```python
from build123d import *

# Parameters (mm, degrees)
F0_R      = 8.5
F1_DEPTH  = 20
F2_W      = 14.2
F2_H      = 5.2
F3_DEPTH  = 15.001
F5_DEPTH  = 15
F6_W      = 1
F6_H      = 2.6394567484
F7_DEPTH  = 20.001
F8_W      = 1.5
F8_H      = 3.5
F9_DEPTH  = 20
F11_DEPTH = 20
F13_DEPTH = 15
F15_DEPTH = 15.001
F16_R     = 3
F17_R     = 0.2
F19_DEPTH = 15


with BuildPart() as f1:
    # F0 (on Front) → F1 (new body)
    with BuildSketch(Plane.XZ):
        with BuildLine():
            Line((0, 18), (0, 0))
            Line((0, 0), (15, 0))
            Line((15, 0), (15, 9.3397459622))
            ThreePointArc((15, 9.3397459622), (15, 26.6602540378), (0, 18))
        make_face()
        with Locations((10, 18)):
            Circle(F0_R, mode=Mode.SUBTRACT)
    extrude(amount=F1_DEPTH)

    # F2 (on face) → F3 (cut, through all)
    with BuildSketch(Plane.YZ.offset(15)):
        Polygon((-3.8, 2), (-2, 2), (-2, 9), (-20, 9), (-20, 7.2), (-3.8, 7.2), align=None)
        with Locations((-12.9, 2.6)):
            Rectangle(F2_W, F2_H)
    extrude(amount=-F3_DEPTH, mode=Mode.SUBTRACT)

    # F4 (on face) → F5 (join, through all)
    with BuildSketch(Plane.YZ.offset(15)):
        Polygon((-20, 7.2), (-15.5, 7.2), (-15.5, 8), align=None)
        Polygon((-15.5, 8.2), (-15.5, 9), (-20, 9), align=None)
    extrude(amount=-F5_DEPTH)

    # F6 (on face) → F7 (cut, through all)
    with BuildSketch(Plane.XZ.offset(20)):
        with Locations((15.5, 10.6594743364)):
            Rectangle(F6_W, F6_H)
    extrude(amount=-F7_DEPTH, mode=Mode.SUBTRACT)

    # F8 (on face) → F9 (join, through all)
    with BuildSketch(Plane.XZ.offset(20)):
        with Locations((14.25, 11.8130682288)):
            Rectangle(F8_W, F8_H)
        Polygon((18.0472665318, 12.0635447138), (16, 11.9792027106), (18, 10), align=None)
    extrude(amount=-F9_DEPTH)

    # F10 (on face) → F11 (cut, through all)
    with BuildSketch(Plane.XZ.offset(20)):
        Polygon((16, 11.9792027106), (16, 10), (17.0662110755, 10), (17.0662110755, 10.9240787853), align=None)
        Polygon((15, 13.5630682288), (13.5, 13.5630682288), (15, 13.0630682288), align=None)
    extrude(amount=-F11_DEPTH, mode=Mode.SUBTRACT)

    # F12 (on face) → F13 (join, through all)
    with BuildSketch(Plane.YZ.offset(15)):
        with BuildLine():
            Line((0, 2), (-5.8, 2))
            ThreePointArc((-5.8, 2), (-2.9, -2.06757233), (0, 2))
        make_face()
    extrude(amount=-F13_DEPTH)

    # F14 (on face) → F15 (cut, through all)
    with BuildSketch(Plane.YZ.offset(15)):
        with BuildLine():
            Line((-2, 2), (-3.8, 2))
            ThreePointArc((-3.8, 2), (-2.9, -0.723853077), (-2, 2))
        make_face()
        with BuildLine():
            Line((0, 2), (0, 9))
            ThreePointArc((0, 9), (-0.3, 5.5), (0, 2))
        make_face()
    extrude(amount=-F15_DEPTH, mode=Mode.SUBTRACT)

    # F16
    f16_edges = [f1.edges().sort_by_distance(p)[0] for p in [
        (7.5, -3.8, 7.2),
        (7.5, -5.8, 5.2),
        (7.5, -3.8, 2),
        (7.5, -2, 2),
        (7.5, 0, 2),
        (7.5, 0, 9),
    ]]
    fillet(f16_edges, radius=F16_R)

    # F17
    f17_edges = [f1.edges().sort_by_distance(p)[0] for p in [
        (7.5, -20, 7.2),
        (7.5, -20, 9),
        (7.5, -15.5, 8.2),
        (7.5, -15.5, 8),
        (7.5, -2, 9),
        (18, -10, 10),
        (16, -10, 11.979203),
        (13.5, -10, 13.563068),
        (15, -10, 13.063068),
        (13.5, -10, 10.254033),
    ]]
    fillet(f17_edges, radius=F17_R)

    # F18 (on face) → F19 (join, through all)
    with BuildSketch(Plane.YZ.offset(15)):
        with BuildLine():
            Line((-2.2, 9), (-15.5, 9))
            ThreePointArc((-15.5, 9), (-8.85, 8.6), (-2.2, 9))
        make_face()
        with BuildLine():
            Line((-15.5, 7.2), (-6.8, 7.2))
            ThreePointArc((-6.8, 7.2), (-11.15, 7.6), (-15.5, 7.2))
        make_face()
        with BuildLine():
            Line((-1.5938824883, 1.5457121977), (-2, 8.8))
            ThreePointArc((-2, 8.8), (-2.381934709, 5.1401063518), (-1.5938824883, 1.5457121977))
        make_face()
    extrude(amount=-F19_DEPTH)


solid = f1.part
```
For this review, take the finished solid that the model builds, in its own axes (mm). A direction names the side the tool comes from. Round coordinates to 2 decimals unless told otherwise and drop trailing zeros. Write each loop counter-clockwise with the first axis right and the second up, starting at its lowest first coordinate (ties: lowest second). Pieces come first, ordered by that corner, then holes. Notation, with made-up numbers: (49, 79) - (60, 79) arc R18 cw to (60, 114) - close; hole circle Ø5 at (53.5, -1.75). An arc over 180 degrees is marked (long way). Answer as a JSON object with one key per item and string values.
1. We need section B-B on z = 24.5. Give the boundary of the cut face in (x, y).
Response values:
{"outline": "(2.4, -20) - (4.52, -20) - (4.52, 0) - (2.4, 0) - close; (15.48, -20) - (17.6, -20) - (17.6, 0) - (15.48, 0) - close"}
2. To check wall thickness, follow line 1 along Z through (x, y) = (10, -9.75); line 2 along Z through (x, y) = (10, -6.75); line 3 along X through (y, z) = (-15.5, 18). State the ranges of each line that lie inside material, in increasing order.
Response values:
{"line 1": "z = 5.2 to 7.56, 8.61 to 9.5, 26.5 to 28", "line 2": "z = 4.39 to 7.2, 8.64 to 9.5, 26.5 to 28", "line 3": "x = 0 to 1.5, 18.5 to 20"}
3. Draft analysis for pull direction X (two halves, no side actions). For faces 4 (the face through (14.306, -10.14, 13.295)), 5 (the face through (7.4, -1.84, 2.09)), 6 (the face through (13.375, -9.86, 27.413)), state which applies: +X half, -X half, draft (parallel to the pull), parting line (faces both ways), or undercut.
Response values:
{"face 4": "undercut", "face 5": "draft", "face 6": "parting line"}
4. We need section D-D on y = -2.9. Give the boundary of the cut face in (x, z), then the cut area to 3 significant figures.
Response values:
{"outline": "(0, -2.07) - (15, -2.07) - (15, -0.72) - (0, -0.72) - close; (0, 8.92) - (15, 8.92) - (15, 12.92) arc R0.2 ccw to (14.86, 13.11) - (13.76, 13.48) arc R0.2 ccw to (13.5, 13.29) - (13.5, 10.38) arc R0.2 cw to (13.38, 10.2) arc R8.5 cw (long way) to (16.14, 12.12) arc R0.2 ccw to (16.14, 11.84) - (17.67, 10.33) arc R0.2 ccw to (18.01, 10.46) - (18.05, 12.06) arc R10 ccw (long way) to (0, 18) - close", "area": "119 mm2"}
5. Tool access review of faces 1 (the face through (8, -14, 5.2)), 2 (the face through (7.6, -2.4, 5.8)), 3 (the face through (7.6, -17.76, 7.6)): name each direction out of +Z, -Z, +X, -X, +Y, -Y from which nothing blocks a thin tool from reaching the whole face with its end or side.
Response values:
{"face 1": "-Z, +X, -X, -Y", "face 2": "+X, -X", "face 3": "+X, -X, -Y"}
6. We need section C-C on z = 1. Give the boundary of the cut face in (x, y), then the cut area to 3 significant figures.
Response values:
{"outline": "(0, -5.97) - (15, -5.97) - (15, -4.4) - (0, -4.4) - close; (0, -1.4) - (15, -1.4) - (15, 0.17) - (0, 0.17) - close", "area": "47.2 mm2"}
7. For pin 1 Ø5 at (x, y) = (14.5, -3) entering from +Z; pin 2 Ø7.5 at (y, z) = (-5.5, 3) entering from +X; pin 3 Ø0.9 at (x, z) = (10, 3.5) entering from +Y, all flat-tipped, find the tip position at first contact; note any pin that passes through.
Response values:
{"pin 1": "stops at z = 27.8", "pin 2": "stops at x = 15", "pin 3": "stops at y = -0.15"}
8. We need section A-A on y = -10.5. Give the boundary of the cut face in (x, z).
Response values:
{"outline": "(0, 5.2) - (15, 5.2) - (15, 7.59) - (0, 7.59) - close; (0, 8.62) - (15, 8.62) - (15, 12.92) arc R0.2 ccw to (14.86, 13.11) - (13.76, 13.48) arc R0.2 ccw to (13.5, 13.29) - (13.5, 10.38) arc R0.2 cw to (13.38, 10.2) arc R8.5 cw (long way) to (16.14, 12.12) arc R0.2 ccw to (16.14, 11.84) - (17.67, 10.33) arc R0.2 ccw to (18.01, 10.46) - (18.05, 12.06) arc R10 ccw (long way) to (0, 18) - close"}
